from build123d import *

# Parameters (mm, degrees)
F0_R     = 10
F0_R_2   = 20
F1_DEPTH = 25


with BuildPart() as f1:
    # F0 (on Top) → F1 (new body)
    with BuildSketch(Plane.XY):
        with BuildLine():
            Line((72.805556, 42.40408), (-51.194444, 42.40408))
            Line((-51.194444, 42.40408), (-51.194444, -40.59592))
            Line((-51.194444, -40.59592), (10.805556, -40.59592))
            ThreePointArc((10.805556, -40.59592), (21.412157, -44.989319), (25.805556, -55.59592))
            Line((25.805556, -55.59592), (25.805556, -60.59592))
            Line((25.805556, -60.59592), (72.805556, -60.59592))
            Line((72.805556, -60.59592), (72.805556, 42.40408))
        make_face()
        with Locations((-21.194444, -22.59592)):
            Circle(F0_R, mode=Mode.SUBTRACT)
        with Locations((48.805556, -27.59592)):
            Circle(F0_R_2, mode=Mode.SUBTRACT)
        with BuildLine():
            Line((-3.194444, 28.40408), (59.805556, 28.40408))
            ThreePointArc((59.805556, 28.40408), (65.46241, 26.060934), (67.805556, 20.40408))
            ThreePointArc((67.805556, 20.40408), (65.46241, 14.747225), (59.805556, 12.40408))
            Line((59.805556, 12.40408), (-3.194444, 12.40408))
            ThreePointArc((-3.194444, 12.40408), (-8.851299, 14.747225), (-11.194444, 20.40408))
            ThreePointArc((-11.194444, 20.40408), (-8.851299, 26.060934), (-3.194444, 28.40408))
        make_face(mode=Mode.SUBTRACT)
    extrude(amount=F1_DEPTH)


solid = f1.part
Verification items for the finished model (mm, model axes). A direction names the side the tool comes from. Round coordinates to 2 decimals unless told otherwise and drop trailing zeros. Loops run counter-clockwise (first coordinate to the right, second up) from the corner with the lowest first, then second, coordinate; pieces in that order, holes last. Notation, with made-up numbers: M 6.25,34.25 L 32.25,34.25 A27 ccw 32.25,63.25 Z; hole C 66.25,-32.75 d7. An arc over 180 degrees is marked long. Write each question's results on one line, items separated by ' | '.
1) Section check C-C on x = 54.5. Record the boundary of the cut face in (y, z), then the cut area to 3 significant figures.
Checks:
outline: M -60.6,0 L -46.77,0 L -46.77,25 L -60.6,25 Z; M -8.42,0 L 12.4,0 L 12.4,25 L -8.42,25 Z; M 28.4,0 L 42.4,0 L 42.4,25 L 28.4,25 Z | area: 1,220 mm2
2) Scan lines: L1, parallel to X at y = -22, z = 19; L2, parallel to Y at x = 27, z = 21.75; L3, parallel to X at y = -18, z = 7.25. Record each from-to range of solid material in increasing order. Write a range as from..to.
Checks:
L1: x = -51.19..-31.18, -11.21..29.6, 68.01..72.81 | L2: y = -60.6..12.4, 28.4..42.4 | L3: x = -51.19..-30.08, -12.31..31.26, 66.35..72.81
3) Mould release check, pull along X, two halves, no side actions. Record for faces 1 (the flat face through (28, 28.404, 12)), 2 (the flat face through (49, -60.596, 12)), 3 (the cylindrical face through (21.29, -44.87, 12.32)): released by +X, released by -X, zero draft, split by the parting line, or undercut.
Checks:
face 1: undercut | face 2: zero draft | face 3: released by -X
4) Section check B-B on y = -14. Record the boundary of the cut face in (x, z).
Checks:
outline: M -51.19,0 L -26.3,0 L -26.3,25 L -51.19,25 Z; M -16.08,0 L 34.14,0 L 34.14,25 L -16.08,25 Z; M 63.47,0 L 72.81,0 L 72.81,25 L 63.47,25 Z
5) Section check D-D on z = 15. Record the boundary of the cut face in (x, y), then the cut area to 3 significant figures.
Checks:
outline: M -51.19,-40.6 L 10.81,-40.6 A15 cw 25.81,-55.6 L 25.81,-60.6 L 72.81,-60.6 L 72.81,42.4 L -51.19,42.4 Z; hole C -21.19,-22.6 d20; hole M -11.19,20.4 A8 ccw -3.19,12.4 L 59.81,12.4 A8 ccw 67.81,20.4 A8 ccw 59.81,28.4 L -3.19,28.4 A8 ccw Z; hole C 48.81,-27.6 d40 | area: 8,500 mm2
6) Section check A-A on x = 3.5. Record the boundary of the cut face in (y, z).
Checks:
outline: M -40.6,0 L 12.4,0 L 12.4,25 L -40.6,25 Z; M 28.4,0 L 42.4,0 L 42.4,25 L 28.4,25 Z
7) Gauge pin test, flat ends, axial feed: P1, Ø12.5, axis at x = -31.5, z = 12.5, coming from the -Y side; P2, Ø4, axis at y = -58, z = 18, coming from the -X side. Record the tip position at first contact, or that the pin passes through.
Checks:
P1: stops at y = -40.6 | P2: stops at x = 25.81
8) Access from +Z, -Z, +X, -X, +Y, -Y to the whole of each face (thin tool, end or side, straight path). Record for faces 4 (the flat face through (-21, -40.596, 12)), 5 (the flat face through (29, 12.404, 12)), 6 (the flat face through (-51.194, 1, 12)).
Checks:
face 4: +Z, -Z, -X, -Y | face 5: +Z, -Z | face 6: +Z, -Z, -X, +Y, -Y
